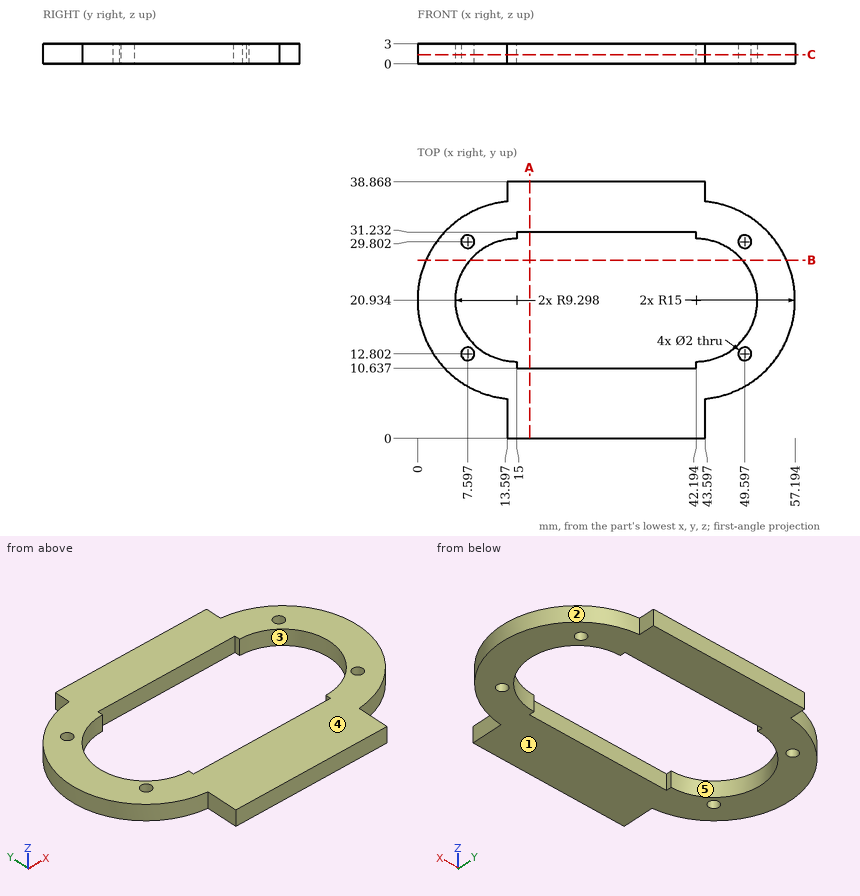
Check sheet for the drawn part. Datum: minimum x, y, z corner. Units: mm. A direction names the side the tool comes from. Round coordinates to 2 decimals unless told otherwise and drop trailing zeros. Order: outer loops, then holes, each group sorted by start corner. A loop starts at its lowest first (then second) coordinate and runs counter-clockwise, first axis right, second up. Notation, with made-up numbers: M 75,39 L 101,39 A28 ccw 101,61 Z; hole C 38.25,28.25 d11. An arc over 180 degrees is marked long. Answer in a Markdown table with one row per item.
(1) Gauge pin test, flat ends, axial feed: pin 1 (0.8 mm diameter, centred on y = 30.5, z = 1.5, fed in from -X) (1 decimal); pin 2 (0.8 mm diameter, centred on y = 11, z = 1.5, fed in from -X); pin 3 (0.9 mm diameter, centred on y = 37.5, z = 1.5, fed in from +X). Record the tip position at first contact, or that the pin passes through.
Findings:
| item | result |
|---|---|
| pin 1 | stops at x = 3.1 |
| pin 2 | stops at x = 3.42 |
| pin 3 | stops at x = 43.6 |
(2) Section check C-C on z = 1.4. Record the boundary of the cut face in (x, y) (1 decimal).
Findings:
| item | result |
|---|---|
| outline | M 13.6,0 L 43.6,0 L 43.6,6 A15 ccw 43.6,35.9 L 43.6,38.9 L 13.6,38.9 L 13.6,35.9 A15 ccw 13.6,6 Z; hole C 7.6,12.8 d2; hole C 7.6,29.8 d2; hole M 15,10.6 L 42.2,10.6 L 42.2,11.6 A9.3 ccw 42.2,30.2 L 42.2,31.2 L 15,31.2 L 15,30.2 A9.3 ccw 15,11.6 Z; hole C 49.6,12.8 d2; hole C 49.6,29.8 d2 |
(3) Section check B-B on y = 27. Record the boundary of the cut face in (x, z).
Findings:
| item | result |
|---|---|
| outline | M 1.28,0 L 7.95,0 L 7.95,3 L 1.28,3 Z; M 49.24,0 L 55.91,0 L 55.91,3 L 49.24,3 Z |
(4) Material ranges on line 1 along Y through (x, z) = (20.5, 2.5); line 2 along X through (y, z) = (27.5, 1.75) (1 decimal); line 3 along Y through (x, z) = (43, 1.3), recorded low to high. Write a range as from..to.
Findings:
| item | result |
|---|---|
| line 1 | y = 0..10.64, 31.23..38.87 |
| line 2 | x = 1.5..8.4, 48.8..55.7 |
| line 3 | y = 0..11.67, 30.2..38.87 |
(5) Set-up check for the marked faces 4 and 5: record each of +Z, -Z, +X, -X, +Y, -Y from which the full face is reachable in a straight line by a thin tool's end or side.
Findings:
| item | result |
|---|---|
| face 4 | +Z, +X, -X, +Y, -Y |
| face 5 | +Z, -Z |
(6) Section check A-A on x = 17. Record the boundary of the cut face in (y, z).
Findings:
| item | result |
|---|---|
| outline | M 0,0 L 10.64,0 L 10.64,3 L 0,3 Z; M 31.23,0 L 38.87,0 L 38.87,3 L 31.23,3 Z |
(7) Draft check along Y on the marked faces 1, 2 and 3. Enter one of: +Y half, -Y half, draft (parallel to the pull), parting line (faces both ways), or undercut.
Findings:
| item | result |
|---|---|
| face 1 | draft |
| face 2 | parting line |
| face 3 | undercut |
